Design review of the part built by this model. Coordinates are the model's own, in mm. A direction names the side the tool comes from. Coordinates: 2 decimals unless noted, no trailing zeros. Loops run counter-clockwise (first coordinate to the right, second up) from the corner with the lowest first, then second, coordinate; pieces in that order, holes last.
from build123d import *

# Parameters (mm, degrees)
IZIM1_W                          = 32
IZIM1_H                          = 50
Y_KSEKLIK_EKSTR_ZYON1_DEPTH      = 32
IZIM2_R                          = 1
IZIM2_W                          = 3
IZIM2_H                          = 11.5
KES_EKSTR_ZYON1_DEPTH            = 32
RADYUS2_R                        = 6
IZIM3_R                          = 11
Y_KSEKLIK_EKSTR_ZYON2_DEPTH      = 5
IZIM4_R                          = 5.5
Y_KSEKLIK_EKSTR_ZYON3_DEPTH      = 3
RADYUS3_R                        = 0.5
Y_KSEKLIK_EKSTR_ZYON4_DEPTH      = 13
Y_KSEKLIK_EKSTR_ZYON4_DEPTH_BACK = 13
IZIM5_W                          = 31
IZIM5_H                          = 37.5


with BuildPart() as part:
    # Çizim1 → Yükseklik-Ekstrüzyon1 (new body)
    with BuildSketch(Plane.XY):
        Rectangle(IZIM1_W, IZIM1_H)
    extrude(amount=Y_KSEKLIK_EKSTR_ZYON1_DEPTH)

    # Çizim2 → Kes-Ekstrüzyon1 (cut)
    with BuildSketch(Plane.XY.offset(32)):
        with Locations((-8, -22.5)):
            Circle(IZIM2_R)
        with Locations((-13.5, -17)):
            Circle(IZIM2_R)
        with Locations((-13.5, -9)):
            Circle(IZIM2_R)
        with Locations((-13.5, -1)):
            Circle(IZIM2_R)
        with Locations((-13.5, 7)):
            Circle(IZIM2_R)
        with Locations((-14.5, 19.25)):
            Rectangle(IZIM2_W, IZIM2_H)
    kes_ekstr_zyon1 = extrude(amount=-KES_EKSTR_ZYON1_DEPTH, mode=Mode.SUBTRACT)

    # Aynalama1: Kes-Ekstrüzyon1 across plane
    add(kes_ekstr_zyon1.mirror(Plane(origin=(0, 0, 0), x_dir=(0, 0, 1), z_dir=(1, 0, 0))), mode=Mode.SUBTRACT)

    # Radyus2
    radyus2_edges = [part.edges().sort_by_distance(p)[0] for p in [
        (-13, 25, 16),
        (13, 25, 16),
    ]]
    fillet(radyus2_edges, radius=RADYUS2_R)

    # Çizim3 → Yükseklik-Ekstrüzyon2 (add)
    with BuildSketch(Plane.XY.offset(32)):
        with Locations((0, 13.5)):
            Circle(IZIM3_R)
    extrude(amount=Y_KSEKLIK_EKSTR_ZYON2_DEPTH)

    # Çizim4 → Yükseklik-Ekstrüzyon3 (add)
    with BuildSketch(Plane(origin=(0, 0, 0), x_dir=(-1, 0, 0), z_dir=(0, 0, -1))):
        with Locations(Location((0, 13.5, 0), (0, 0, 180))):
            Circle(IZIM4_R)
    extrude(amount=Y_KSEKLIK_EKSTR_ZYON3_DEPTH)

    # Radyus3
    radyus3_edges = [part.edges().sort_by_distance(p)[0] for p in [
        (-5.5, 13.5, 0),
        (0, -25, 32),
        (-16, -5.75, 0),
        (-16, -5.75, 32),
        (-13, 16.25, 0),
        (-14.5, 13.5, 0),
        (-13, 13.5, 16),
        (-16, 13.5, 16),
        (-14.5, 13.5, 32),
        (-13, 16.25, 32),
        (16, -5.75, 32),
        (0, -25, 0),
        (16, -5.75, 0),
        (14.5, 13.5, 32),
        (16, 13.5, 16),
        (13, 16.25, 32),
        (13, 13.5, 16),
        (14.5, 13.5, 0),
        (13, 16.25, 0),
        (16, -25, 16),
        (-16, -25, 16),
        (0, 25, 32),
        (-11.242640687, 23.242640687, 32),
        (11.242640687, 23.242640687, 32),
        (0, 25, 0),
        (-11.242640687, 23.242640687, 0),
        (11.242640687, 23.242640687, 0),
    ]]
    fillet(radyus3_edges, radius=RADYUS3_R - 0.0001)  # a hair under: the kernel refuses the full size

    # Çizim5 → Yükseklik-Ekstrüzyon4 (add, two sides: drawn at the far end of the back side and taken through both)
    with BuildSketch(Plane.XY.offset(16).offset(-Y_KSEKLIK_EKSTR_ZYON4_DEPTH_BACK)):
        with Locations((0, -5.75)):
            Rectangle(IZIM5_W, IZIM5_H)
    extrude(amount=Y_KSEKLIK_EKSTR_ZYON4_DEPTH + Y_KSEKLIK_EKSTR_ZYON4_DEPTH_BACK)


solid = part.part
Q1. Machinability: for faces 4 (the flat face through (13, -17, 3)), 5 (the cylindrical face through (8.217, -23.476, 30.521)), 6 (the flat face through (-16, -6, 16)), which of the approach directions +Z, -Z, +X, -X, +Y, -Y give a long, thin tool a straight path to every point of the face, cutting with its end or side? Answer none if there is none.
Q2. Take a section at A-A, the plane y = -1. Write out the cut boundary in (x, z), then the cut area to 4 significant figures.
Q3. Clearance check with flat-ended pins moving along their axes: pin 1 Ø1.6 at (x, z) = (-14, 11) entering from +Y; pin 2 Ø5 at (x, y) = (-7, -4.5) entering from -Z; pin 3 Ø0.6 at (x, y) = (-13.5, -16.5) entering from -Z. State where each tip first meets the part, or that it passes through.
Q4. Take a section at C-C, the plane y = -14. Write out the cut boundary in (x, z).
Q5. The part is to be moulded in two halves that separate along X. For faces 1 (the cylindrical face through (-2.38, 2.76, 34.47)), 2 (the cylindrical face through (-11.289, 23.196, 15.783)), 3 (the flat face through (13, -1, 29)), say which applies: pulls with the +X half, pulls with the -X half, needs draft (parallel to the pull), parting line crosses it, or undercut.
Q6. For line 1 (Y direction, x = 13.5, z = 2.05); line 2 (Z direction, x = 7.5, y = -16); line 3 (Z direction, x = -8, y = 12.5), list the stretches that pass through material, from the lowest coordinate up.
Q7. Take a section at B-B, the plane z = 23.5. Write out the cut boundary in (x, y).
Q8. Take a section at D-D, the plane y = 4. Write out the cut boundary in (x, z).
Entries:
1. face 4: -Z
1. face 5: +Z
1. face 6: +Z, -Z, -X, +Y, -Y
2. outline: (-16, 0.5) arc R0.5 ccw to (-15.5, 0) - (-14.5, 0) - (-14.5, 3) - (-12.5, 3) - (-12.5, 0) - (12.5, 0) - (12.5, 3) - (14.5, 3) - (14.5, 0) - (15.5, 0) arc R0.5 ccw to (16, 0.5) - (16, 31.5) arc R0.5 ccw to (15.5, 32) - (14.5, 32) - (14.5, 29) - (12.5, 29) - (12.5, 32) - (-12.5, 32) - (-12.5, 29) - (-14.5, 29) - (-14.5, 32) - (-15.5, 32) arc R0.5 ccw to (-16, 31.5) - close
2. area: 1,000 mm2
3. pin 1: stops at y = 13.6
3. pin 2: stops at z = 0
3. pin 3: stops at z = 3
4. outline: (-16, 0.5) arc R0.5 ccw to (-15.5, 0) - (15.5, 0) arc R0.5 ccw to (16, 0.5) - (16, 31.5) arc R0.5 ccw to (15.5, 32) - (-15.5, 32) arc R0.5 ccw to (-16, 31.5) - close
5. face 1: parting line crosses it
5. face 2: pulls with the -X half
5. face 3: undercut
6. line 1: y = -25 to -18, -16 to -10, -8 to -2, 0 to 6, 8 to 13.5
6. line 2: z = 0 to 32
6. line 3: z = 0 to 37
7. outline: (-16, -24.5) arc R0.5 ccw to (-15.5, -25) - (15.5, -25) arc R0.5 ccw to (16, -24.5) - (16, 13) arc R0.5 ccw to (15.5, 13.5) - (13.5, 13.5) arc R0.5 cw to (13, 14) - (13, 19) arc R6 ccw to (7, 25) - (-7, 25) arc R6 ccw to (-13, 19) - (-13, 14) arc R0.5 cw to (-13.5, 13.5) - (-15.5, 13.5) arc R0.5 ccw to (-16, 13) - close
8. outline: (-16, 0.5) arc R0.5 ccw to (-15.5, 0) - (15.5, 0) arc R0.5 ccw to (16, 0.5) - (16, 31.5) arc R0.5 ccw to (15.5, 32) - (5.55, 32) - (5.55, 37) - (-5.55, 37) - (-5.55, 32) - (-15.5, 32) arc R0.5 ccw to (-16, 31.5) - close
